from build123d import *

# Parameters (mm, degrees)
SKETCH1_R                = 25
SKETCH1_R_2              = 20
BOSS_EXTRUDE1_DEPTH      = 20
SKETCH1_W                = 70
SKETCH1_H                = 10
BOSS_EXTRUDE1_2_DEPTH    = 20
BOSS_EXTRUDE2_DEPTH      = 50
BOSS_EXTRUDE2_DEPTH_BACK = 20
SKETCH1_4_W              = 70
SKETCH1_4_H              = 10
BOSS_EXTRUDE3_DEPTH      = 25
BOSS_EXTRUDE3_DEPTH_BACK = 20
SKETCH1_5_R              = 20
SKETCH1_5_R_2            = 15
FILLET1_R                = 20
CUT_EXTRUDE1_DEPTH       = 161.623784042


with BuildPart() as part:
    # Sketch1 → Boss-Extrude1 (new body)
    with BuildSketch(Plane.XY):
        with BuildLine():
            Line((0, 60), (0, 20))
            Line((0, 20), (70, 20))
            Line((70, 20), (70, 25))
            ThreePointArc((70, 25), (77.32233047, 42.67766953), (95, 50))
            Line((95, 50), (105, 50))
            ThreePointArc((105, 50), (130, 75), (105, 100))
            Line((105, 100), (40, 100))
            ThreePointArc((40, 100), (11.715728753, 88.284271247), (0, 60))
        make_face()
        with Locations((40, 60)):
            Circle(SKETCH1_R, mode=Mode.SUBTRACT)
        with Locations((105, 75)):
            Circle(SKETCH1_R_2, mode=Mode.SUBTRACT)
    extrude(amount=-BOSS_EXTRUDE1_DEPTH)



with BuildPart() as body_2:
    # Sketch1 → Boss-Extrude1 2 (new body)
    with BuildSketch(Plane.XY):
        with Locations((35, 5)):
            Rectangle(SKETCH1_W, SKETCH1_H)
    extrude(amount=-BOSS_EXTRUDE1_2_DEPTH)


with BuildPart() as part_1:
    add(part.part)

    add(body_2.part)  # Boss-Extrude2 merges body 2
    # Sketch1<4> → Boss-Extrude2 (add, two sides: drawn at the far end of the back side and taken through both)
    with BuildSketch(Plane.XY.offset(-BOSS_EXTRUDE2_DEPTH_BACK)):
        with Locations((35, 15)):
            Rectangle(SKETCH1_4_W, SKETCH1_4_H)
    extrude(amount=BOSS_EXTRUDE2_DEPTH + BOSS_EXTRUDE2_DEPTH_BACK)

    # Sketch1<5> → Boss-Extrude3 (add, two sides: drawn at the far end of the back side and taken through both)
    with BuildSketch(Plane.XY.offset(-BOSS_EXTRUDE3_DEPTH_BACK)):
        with Locations((105, 75)):
            Circle(SKETCH1_5_R)
        with Locations((105, 75)):
            Circle(SKETCH1_5_R_2, mode=Mode.SUBTRACT)
    extrude(amount=BOSS_EXTRUDE3_DEPTH + BOSS_EXTRUDE3_DEPTH_BACK)

    # Fillet1
    fillet1_edges = [part_1.edges().sort_by_distance(p)[0] for p in [
        (70, 15, 50),
        (0, 15, 50),
    ]]
    fillet(fillet1_edges, radius=FILLET1_R)

    # Sketch2 → Cut-Extrude1 (cut, through all)
    with BuildSketch(Plane(origin=(0, 20, 0), x_dir=(1, 0, 0), z_dir=(0, 1, 0))):
        with BuildLine():
            Line((20, -15), (50, -15))
            ThreePointArc((50, -15), (65, -30), (50, -45))
            Line((50, -45), (20, -45))
            ThreePointArc((20, -45), (5, -30), (20, -15))
        make_face()
    extrude(amount=-CUT_EXTRUDE1_DEPTH, mode=Mode.SUBTRACT)


solid = part_1.part
Work out the finished part from the listing and answer in its coordinate system (mm). A direction names the side the tool comes from. Coordinates: 2 decimals unless noted, no trailing zeros. Write each loop counter-clockwise with the first axis right and the second up, starting at its lowest first coordinate (ties: lowest second). Pieces come first, ordered by that corner, then holes.
1. The part is cut by section A-A, the plane x = 47. Write down the section's boundary in (y, z), and give its area (3 significant figures).
Results list:
outline: (0, -20) - (36, -20) - (36, 0) - (20, 0) - (20, 15) - (10, 15) - (10, 0) - (0, 0) - close; (10, 45) - (20, 45) - (20, 50) - (10, 50) - close; (84, -20) - (100, -20) - (100, 0) - (84, 0) - close
area: 1,240 mm2
2. The part is cut by section B-B, the plane z = -15. Write down the section's boundary in (x, y).
Results list:
outline: (0, 0) - (70, 0) - (70, 25) arc R25 cw to (95, 50) - (105, 50) arc R25 ccw to (105, 100) - (40, 100) arc R40 ccw to (0, 60) - close; hole circle Ø50 at (40, 60); hole circle Ø30 at (105, 75)
3. The part is cut by section D-D, the plane y = 83. Write down the section's boundary in (x, z), and give its area (3 significant figures).
Results list:
outline: (7.27, -20) - (30.2, -20) - (30.2, 0) - (7.27, 0) - close; (49.8, -20) - (92.31, -20) - (92.31, 25) - (86.67, 25) - (86.67, 0) - (49.8, 0) - close; (117.69, -20) - (128.69, -20) - (128.69, 0) - (123.33, 0) - (123.33, 25) - (117.69, 25) - close
area: 1,810 mm2
4. For faces 1 (the flat face through (35, 10, 14)), 2 (the cylindrical face through (89, 63, 12)), 3 (the flat face through (35, 15, 45)), 4 (the flat face through (100, 50, -10)), determine the directions among +Z, -Z, +X, -X, +Y, -Y from which every point of the face is accessible in a straight line to the end or side of a thin tool.
Results list:
face 1: +Z, +X, -X, -Y
face 2: +Z
face 3: +Y, -Y
face 4: +Z, -Z, +X, -Y
5. For a pull along X with two mould halves and no side action, classify faces 5 (the cylindrical face through (129.994, 74.45, -9.86)), 6 (the cylindrical face through (101.748, 60.357, 2.185)), 7 (the flat face through (108, 90, 25)) as +X half, -X half, draft (parallel to the pull), parting line (faces both ways), or undercut.
Results list:
face 5: +X half
face 6: undercut
face 7: draft
6. Flat-ended cylindrical pins translate along their axes: pin 1 (12.5 mm diameter, centred on y = 8, z = 8, fed in from +X); pin 2 (12 mm diameter, centred on x = 99.5, y = 75, fed in from -Z); pin 3 (2 mm diameter, centred on y = 66.5, z = 15.5, fed in from +X); pin 4 (10 mm diameter, centred on y = 57.5, z = 3, fed in from +X). Find the tip coordinate at first contact, or state that the pin passes through.
Results list:
pin 1: stops at x = 70
pin 2: passes through
pin 3: stops at x = 123.54
pin 4: stops at x = 126.04
7. The part is cut by section C-C, the plane y = 47. Write down the section's boundary in (x, z), and give its area (3 significant figures).
Results list:
outline: (0, -20) - (18.65, -20) - (18.65, 0) - (0, 0) - close; (61.35, -20) - (83.13, -20) - (83.13, 0) - (61.35, 0) - close
area: 808 mm2
8. Consider line 1 along Y through (x, z) = (105, 12); line 2 along X through (y, z) = (83, -0.5); line 3 along Y through (x, z) = (40, -10.5). Determine where each line is inside the solid, lowest interval first.
Results list:
line 1: y = 55 to 60, 90 to 95
line 2: x = 7.27 to 30.2, 49.8 to 92.31, 117.69 to 128.69
line 3: y = 0 to 35, 85 to 100
